Read the model definition and answer for the solid it produces. Units are mm, in the model's axes. Face numbers are marked on the shaded views. A direction names the side the tool comes from. Round coordinates to 2 decimals unless told otherwise and drop trailing zeros. Order: outer loops, then holes, each group sorted by start corner. A loop starts at its lowest first (then second) coordinate and runs counter-clockwise, first axis right, second up.
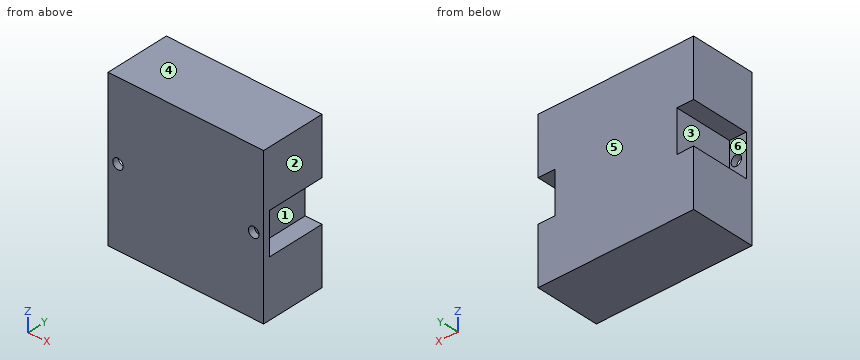
from build123d import *

# Parameters (mm, degrees)
SKETCH_1_W          = 74.5
SKETCH_1_H          = 74.5
EXTRUDE_1_DEPTH     = 31
SKETCH_2_W          = 8
SKETCH_2_H          = 20
CUT_EXTRUDE_1_DEPTH = 28
SKETCH_3_R          = 2.5
CUT_EXTRUDE_2_DEPTH = 60.658402593


with BuildPart() as part:
    # 草图1 → 凸台-拉伸1 (new body)
    with BuildSketch(Plane(origin=(0, 0, 0), x_dir=(1, 0, 0), z_dir=(0, 1, 0))):
        Rectangle(SKETCH_1_W, SKETCH_1_H)
    extrude(amount=EXTRUDE_1_DEPTH)

    # 草图2 → 切除-拉伸1 (cut)
    with BuildSketch(Plane(origin=(0, 31, 0), x_dir=(1, 0, 0), z_dir=(0, 1, 0))):
        with Locations((-33.25, 0)):
            Rectangle(SKETCH_2_W, SKETCH_2_H)
        with Locations((33.25, 0)):
            Rectangle(SKETCH_2_W, SKETCH_2_H)
    extrude(amount=-CUT_EXTRUDE_1_DEPTH, mode=Mode.SUBTRACT)

    # 草图3 → 切除-拉伸2 (cut, through all)
    with BuildSketch(Plane(origin=(0, 3, 0), x_dir=(1, 0, 0), z_dir=(0, 1, 0))):
        with Locations(Location((-32.5, 0, 0), (0, 0, 270))):
            Circle(SKETCH_3_R)
        with Locations(Location((32.5, 0, 0), (0, 0, 270))):
            Circle(SKETCH_3_R)
    extrude(amount=-CUT_EXTRUDE_2_DEPTH, mode=Mode.SUBTRACT)


solid = part.part
Q1. A cutting plane is placed at D-D, the plane y = 14. Give the vertices of the cut face in (x, z), plus the area to 3 significant figures.
Outcome:
outline: (-37.25, -37.25) - (37.25, -37.25) - (37.25, -10) - (29.25, -10) - (29.25, 10) - (37.25, 10) - (37.25, 37.25) - (-37.25, 37.25) - (-37.25, 10) - (-29.25, 10) - (-29.25, -10) - (-37.25, -10) - close
area: 5,230 mm2
Q2. A cutting plane is placed at C-C, the plane z = 0. Give the vertices of the cut face in (x, y).
Outcome:
outline: (-37.25, 0) - (-35, 0) - (-35, 3) - (-37.25, 3) - close; (-30, 0) - (30, 0) - (30, 3) - (29.25, 3) - (29.25, 31) - (-29.25, 31) - (-29.25, 3) - (-30, 3) - close; (35, 0) - (37.25, 0) - (37.25, 3) - (35, 3) - close
Q3. For a pull along Z with two mould halves and no side action, classify the marked faces 1, 2, 3 and 4 as released by +Z, released by -Z, zero draft, split by the parting line, or undercut.
Outcome:
face 1: undercut
face 2: zero draft
face 3: undercut
face 4: released by +Z
Q4. A cutting plane is placed at B-B, the plane x = -32.5. Give the vertices of the cut face in (y, z), plus the area to 3 significant figures.
Outcome:
outline: (0, -37.25) - (31, -37.25) - (31, -10) - (3, -10) - (3, -2.5) - (0, -2.5) - close; (0, 2.5) - (3, 2.5) - (3, 10) - (31, 10) - (31, 37.25) - (0, 37.25) - close
area: 1,730 mm2
Q5. For the marked faces 5 and 6, determine the directions among +Z, -Z, +X, -X, +Y, -Y from which every point of the face is accessible in a straight line to the end or side of a thin tool.
Outcome:
face 5: +Z, -Z, +X, -X, +Y
face 6: -X, +Y
Q6. Straight lines are drawn through the part: probe 1 along X at (y, z) = (0.85, 0); probe 2 along Z at (x, y) = (-30, 23); probe 3 along Y at (x, z) = (-30.5, 3.5). For each, find the intervals that lie inside material, in ascending order.
Outcome:
probe 1: x = -37.25 to -35, -30 to 30, 35 to 37.25
probe 2: z = -37.25 to -10, 10 to 37.25
probe 3: y = 0 to 3
Q7. Flat-ended cylindrical pins translate along their axes: pin 1 (10 mm diameter, centred on y = 16.5, z = 1.5, fed in from +X); pin 2 (8 mm diameter, centred on x = 32.5, z = 0, fed in from -Y); pin 3 (2.5 mm diameter, centred on x = -34, z = 3.5, fed in from +Y). Find the tip coordinate at first contact, or state that the pin passes through.
Outcome:
pin 1: stops at x = 29.25
pin 2: stops at y = 0
pin 3: stops at y = 3
Q8. A cutting plane is placed at A-A, the plane z = 9. Give the vertices of the cut face in (x, y).
Outcome:
outline: (-37.25, 0) - (37.25, 0) - (37.25, 3) - (29.25, 3) - (29.25, 31) - (-29.25, 31) - (-29.25, 3) - (-37.25, 3) - close
